```python
from build123d import *

# Parameters (mm, degrees)
F1_DEPTH = 14
F2_R     = 0.99999
F3_SIZE  = 0.5
F4_R     = 2


# Not quite as in the source:
# - a fillet or chamfer is up to 0.001 mm smaller than in the source, because OpenCascade refuses the exact size


with BuildPart() as f1:
    # F0 (on Front) → F1 (new body)
    with BuildSketch(Plane.XZ):
        with BuildLine():
            Line((-68.4901475161, 21), (-167.4901475161, 21))
            Line((-167.4901475161, 21), (-167.4901475161, 0))
            Line((-167.4901475161, 0), (-149.4901475161, 0))
            Line((-149.4901475161, 0), (-149.4901475161, 2))
            Line((-149.4901475161, 2), (-165.4901475161, 2))
            Line((-165.4901475161, 2), (-165.4901475161, 19))
            Line((-165.4901475161, 19), (-70.4901475161, 19))
            Line((-70.4901475161, 19), (-70.4901475161, 2))
            Line((-70.4901475161, 2), (-86.4901475161, 2))
            Line((-86.4901475161, 2), (-86.4901475161, 0))
            Line((-86.4901475161, 0), (-68.4901475161, 0))
            Line((-68.4901475161, 0), (-68.4901475161, 19))
            Line((-68.4901475161, 19), (16.5098524839, 19))
            Line((16.5098524839, 19), (16.5098524839, 21))
            Line((16.5098524839, 21), (16.5098524839, 31))
            Line((16.5098524839, 31), (14.5098524839, 31))
            ThreePointArc((14.5098524839, 31), (13.7436966654, 25.7798467455), (11.5098524839, 21))
            Line((11.5098524839, 21), (-63.147776881, 21))
            Line((-63.147776881, 21), (-68.4901475161, 21))
        make_face()
    extrude(amount=F1_DEPTH)

    # F2 (radius 1 in the source; OpenCascade refuses exactly that, so slightly less here)
    f2_edges = [f1.edges().sort_by_distance(p)[0] for p in [
        (14.509852, -7, 31),
        (16.509852, -7, 31),
        (16.509852, -7, 19),
        (-70.490148, -7, 2),
        (-70.490148, -7, 19),
        (-86.490148, -7, 2),
        (-86.490148, -7, 0),
        (-68.490148, -7, 0),
        (-165.490148, -7, 19),
        (-149.490148, -7, 2),
        (-167.490148, -7, 0),
        (-167.490148, -7, 21),
    ]]
    fillet(f2_edges, radius=F2_R)

    # F3
    f3_edges = [f1.edges().sort_by_distance(p)[0] for p in [
        (-77.490153, 0, 21),
        (-117.990148, 0, 19),
        (-167.490148, -14, 10.5),
        (-68.490148, -14, 9.999995),
    ]]
    chamfer(f3_edges, length=F3_SIZE)

    # F4
    f4_edges = [f1.edges().sort_by_distance(p)[0] for p in [
        (11.509852, -7, 21),
    ]]
    fillet(f4_edges, radius=F4_R)


solid = f1.part
```
Verification items for the finished model (mm, model axes). A direction names the side the tool comes from. Round coordinates to 2 decimals unless told otherwise and drop trailing zeros. Order: outer loops, then holes, each group sorted by start corner. A loop starts at its lowest first (then second) coordinate and runs counter-clockwise, first axis right, second up.
1) Cross-section at D-D, the plane x = -108.5. Record the cut outline in (y, z), plus the area to 3 significant figures.
Geometry says:
outline: (-14, 19.5) - (-13.5, 19) - (-0.5, 19) - (0, 19.5) - (0, 20.5) - (-0.5, 21) - (-13.5, 21) - (-14, 20.5) - close
area: 27.5 mm2
2) Cross-section at B-B, the plane x = -155. Record the cut outline in (y, z).
Geometry says:
outline: (-14, 0.5) - (-13.5, 0) - (-0.5, 0) - (0, 0.5) - (0, 2) - (-14, 2) - close; (-14, 19.5) - (-13.5, 19) - (-0.5, 19) - (0, 19.5) - (0, 20.5) - (-0.5, 21) - (-13.5, 21) - (-14, 20.5) - close
3) Draft check along X on faces 1 (the cylindrical face through (13.863, -6.902, 26.196)), 2 (the flat face through (-119, -7, 19)), 3 (the flat face through (-62.1, 0, 19.2)), 4 (the flat face through (16.51, -7, 25)). Enter one of: +X half, -X half, draft (parallel to the pull), parting line (faces both ways), or undercut.
Geometry says:
face 1: -X half
face 2: undercut
face 3: draft
face 4: +X half
4) Depth check by flat-ended pin: pin 1 (4 mm diameter, centred on x = -134.5, y = -3.5, fed in from -Z); pin 2 (4 mm diameter, centred on y = -5, z = 9, fed in from +X); pin 3 (1 mm diameter, centred on x = -123, y = -8, fed in from +Z). Enter the tip coordinate at first touch or a pass-through.
Geometry says:
pin 1: stops at z = 19
pin 2: stops at x = -68.49
pin 3: stops at z = 21
5) Material ranges on line 1 (X direction, y = -8.25, z = 10.5); line 2 (Z direction, x = -83, y = -7.25); line 3 (Z direction, x = -19, y = -10.5), recorded low to high.
Geometry says:
line 1: x = -167.49 to -165.49, -70.49 to -68.49
line 2: z = 0 to 2, 19 to 21
line 3: z = 19 to 21
6) Tool access check on faces 5 (the flat face through (-78, -7, 0)), 6 (the flat face through (-62.1, -14, 19.2)), 7 (the flat face through (-78, -7, 2)), 8 (the flat face through (-77, -7, 21)), 9 (the flat face through (-27, -7, 19)). Record the directions out of +Z, -Z, +X, -X, +Y, -Y that give a thin tool (end or side, any length) a straight path to the whole face; none if there is none.
Geometry says:
face 5: -Z, +X, -X, +Y, -Y
face 6: +Z, -Z, +X, -X, -Y
face 7: +Y, -Y
face 8: +Z, -X, +Y, -Y
face 9: -Z, +X, +Y, -Y
7) Cross-section at A-A, the plane z = 7. Record the cut outline in (x, y).
Geometry says:
outline: (-167.49, -13.5) - (-166.99, -14) - (-165.99, -14) - (-165.49, -13.5) - (-165.49, -0.5) - (-165.99, 0) - (-166.99, 0) - (-167.49, -0.5) - close; (-70.49, -13.5) - (-69.99, -14) - (-68.99, -14) - (-68.49, -13.5) - (-68.49, -0.5) - (-68.99, 0) - (-69.99, 0) - (-70.49, -0.5) - close
